Could you check a few things on this model? Use its own coordinates, in mm. A direction names the side the tool comes from. Give positions to 0.01 mm unless a question says otherwise; leave off trailing zeros. Loops run counter-clockwise (first coordinate to the right, second up) from the corner with the lowest first, then second, coordinate; pieces in that order, holes last.
1. For faces 4 (the flat face through (0, -1, 0)), 5 (the flat face through (11, 12, 0)), which set-ups out of +Z, -Z, +X, -X, +Y, -Y let a thin tool reach every point of the face, with its end or its side?
2. Imagine slicing it at C-C (z = -18). List the corners of the cut face in (x, y) for me.
3. Imagine slicing it at A-A (z = 13.5). List the corners of the cut face in (x, y) for me, plus the area to 3 significant figures.
4. Thinking about a two-plate mould opening in Z: for faces 1 (the flat face through (-1, -1, 0)), 2 (the flat face through (-0.3, 3.6, -21.5)), 3 (the cylindrical face through (-0.51, -5.69, -12.26)), which applies, +Z half, -Z half, draft (parallel to the pull), parting line (faces both ways), or undercut?
5. I need wall thicknesses on line 1 along Z through (x, y) = (5.08, 11.85); line 2 along X through (y, z) = (5, 7); line 3 along Y through (x, z) = (5.25, 11). Which ranges of each line are inside material? Lowest first, please.
6. Imagine slicing it at B-B (x = 5.5). List the corners of the cut face in (y, z) for me, plus the area to 3 significant figures.
7. For P1, Ø4, axis at y = 9, z = 9.5, coming from the +X side; P2, Ø5, axis at x = 7, z = 0.5, coming from the -Y side; P3, Ø4, axis at y = -5.85, z = 13.5, coming from the +X side, each with a flat end and sliding along its axis, tell me the tip position at first contact or that it passes through.
8. Imagine slicing it at D-D (y = -7.75). List the corners of the cut face in (x, z) for me.
```python
from build123d import *

# Parameters (mm, degrees)
SKETCH1_W                    = 43
SKETCH1_H                    = 25
BASE_FLANGE1_DEPTH           = 1
EDGE_FLANGE1_STRIP_W         = 6
EDGE_FLANGE1_STRIP_H         = 1
EDGE_FLANGE1_STRIP_CUT_DEPTH = 43
EDGE_FLANGE1_DEPTH           = 43
TAP_DRILL_FOR_M3_TAP1_D      = 2.5
TAP_DRILL_FOR_M3_TAP2_D      = 2.5
TAP_DRILL_FOR_M3_TAP2_DEPTH  = 10
TAP_DRILL_FOR_M3_TAP2_TIP    = 0.751075774


# Sheet-metal steps are written as plain solids
with BuildPart() as part:
    # Sketch1 → Base-Flange1 (new body)
    with BuildSketch(Plane(origin=(0, 0, 0), x_dir=(0, 0, -1), z_dir=(1, 0, 0))):
        Rectangle(SKETCH1_W, SKETCH1_H)
    extrude(amount=-BASE_FLANGE1_DEPTH)

    # Edge-Flange1 strip (across the edge) → Edge-Flange1 strip cut (cut)
    with BuildSketch(Plane(origin=(0, 12.5, -21.5), x_dir=(0, -1, 0), z_dir=(0, 0, 1))):
        with Locations((-1, -0.5)):
            Rectangle(EDGE_FLANGE1_STRIP_W, EDGE_FLANGE1_STRIP_H)
    extrude(amount=EDGE_FLANGE1_STRIP_CUT_DEPTH, mode=Mode.SUBTRACT)

    # Edge-Flange1 section (across the edge) → Edge-Flange1 (add)
    with BuildSketch(Plane(origin=(0, 12.5, -21.5), x_dir=(0, -1, 0), z_dir=(0, 0, 1))):
        with BuildLine():
            Line((0, 1), (0, 11))
            Line((0, 11), (1, 11))
            Line((1, 11), (1, 1))
            ThreePointArc((1, 1), (1.292893219, 0.292893219), (2, 0))
            Line((2, 0), (2, -1))
            ThreePointArc((2, -1), (0.585786438, -0.414213562), (0, 1))
        make_face()
    extrude(amount=EDGE_FLANGE1_DEPTH)

    # Tap Drill for M3 Tap1 (through all)
    with Locations(Plane(origin=(-360.471522339, 12.5, -232.457964235), x_dir=(-1, 0, 0), z_dir=(0, 1, 0))):
        with Locations((-365.551522339, 237.387201908), (-365.551522339, 217.887201908)):
            Hole(TAP_DRILL_FOR_M3_TAP1_D / 2)

    # Tap Drill for M3 Tap2
    with Locations(Plane(origin=(2, 426.094482546, -232.457964235), x_dir=(0, 1, 0), z_dir=(1, 0, 0))):
        with Locations((-431.942500863, 218.957964235), (-431.942500863, 245.957964235)):
            Hole(TAP_DRILL_FOR_M3_TAP2_D / 2, depth=TAP_DRILL_FOR_M3_TAP2_DEPTH)
            with Locations((0, 0, -(TAP_DRILL_FOR_M3_TAP2_DEPTH + TAP_DRILL_FOR_M3_TAP2_TIP / 2))):  # 118° drill point
                Cone(0, TAP_DRILL_FOR_M3_TAP2_D / 2, TAP_DRILL_FOR_M3_TAP2_TIP, mode=Mode.SUBTRACT)


solid = part.part
```
Derived:
1. face 4: +Z, -Z, +X, -Y
1. face 5: +Z, -Z, +X, +Y, -Y
2. outline: (-1, -12.5) - (0, -12.5) - (0, 10.5) arc R1 cw to (1, 11.5) - (11, 11.5) - (11, 12.5) - (1, 12.5) arc R2 ccw to (-1, 10.5) - close
3. outline: (-1, -12.5) - (0, -12.5) - (0, -7.1) - (-1, -7.1) - close; (-1, -4.6) - (0, -4.6) - (0, 10.5) arc R1 cw to (1, 11.5) - (11, 11.5) - (11, 12.5) - (1, 12.5) arc R2 ccw to (-1, 10.5) - close
3. area: 32.9 mm2
4. face 1: draft
4. face 2: -Z half
4. face 3: undercut
5. line 1: z = -21.5 to -15.82, -13.32 to 3.68, 6.18 to 21.5
5. line 2: x = -1 to 0
5. line 3: y = 11.5 to 12.5
6. outline: (11.5, -21.5) - (12.5, -21.5) - (12.5, -15.75) - (11.5, -15.75) - close; (11.5, -13.39) - (12.5, -13.39) - (12.5, 3.75) - (11.5, 3.75) - close; (11.5, 6.11) - (12.5, 6.11) - (12.5, 21.5) - (11.5, 21.5) - close
6. area: 38.3 mm2
7. P1: stops at x = 0.13
7. P2: stops at y = 11.5
7. P3: stops at x = 0
8. outline: (-1, -21.5) - (0, -21.5) - (0, 21.5) - (-1, 21.5) - close
